Design review of the part built by this model. Coordinates are the model's own, in mm. Round coordinates to 2 decimals unless told otherwise and drop trailing zeros. Use a Markdown table: item, result.
from build123d import *

# Parameters (mm, degrees)
SKETCH1_W                        = 1212.85
SKETCH1_H                        = 584.2
BOSS_EXTRUDE1_DEPTH              = 3.175
SKETCH2_R                        = 5.3578125
SKETCH2_W                        = 63.5
SKETCH2_H                        = 88.9
CUT_EXTRUDE1_DEPTH               = 674.137439996
FILLET1_R                        = 6.35
SKETCH3_W                        = 142.875
SKETCH3_H                        = 88.9
CUT_EXTRUDE2_DEPTH               = 674.137439996
F_27_64_0_42188_DIAMETER_HOLE1_D = 10.715752
LPATTERN1_COUNT                  = 5
LPATTERN1_PITCH                  = 279.4
CUT_EXTRUDE3_DEPTH               = 674.137439996


with BuildPart() as part:
    # Sketch1 → Boss-Extrude1 (new, symmetric)
    with BuildSketch(Plane.XY):
        Rectangle(SKETCH1_W, SKETCH1_H)
    extrude(amount=BOSS_EXTRUDE1_DEPTH, both=True)

    # Sketch2 → Cut-Extrude1 (cut, through all)
    with BuildSketch(Plane.XY.offset(3.175)):
        with Locations((-466.725, 139.7)):
            Circle(SKETCH2_R)
        with Locations((-409.575, 139.7)):
            Circle(SKETCH2_R)
        with Locations((-466.725, -241.3)):
            Circle(SKETCH2_R)
        with Locations((-409.575, -241.3)):
            Circle(SKETCH2_R)
        with Locations((412.75, 139.7)):
            Circle(SKETCH2_R)
        with Locations((463.55, 139.7)):
            Circle(SKETCH2_R)
        with Locations((412.75, -241.3)):
            Circle(SKETCH2_R)
        with Locations((463.55, -241.3)):
            Circle(SKETCH2_R)
        with Locations((438.15, 247.65)):
            Rectangle(SKETCH2_W, SKETCH2_H)
        with Locations((-438.15, 247.65)):
            Rectangle(SKETCH2_W, SKETCH2_H)
    extrude(amount=-CUT_EXTRUDE1_DEPTH, mode=Mode.SUBTRACT)

    # Fillet1
    fillet1_edges = [part.edges().sort_by_distance(p)[0] for p in [
        (-406.4, 203.2, 0),
        (-469.9, 203.2, 0),
        (469.9, 203.2, 0),
        (406.4, 203.2, 0),
    ]]
    fillet(fillet1_edges, radius=FILLET1_R)

    # Sketch3 → Cut-Extrude2 (cut, through all)
    with BuildSketch(Plane.XY.offset(3.175)):
        with Locations((534.9875, 247.65)):
            Rectangle(SKETCH3_W, SKETCH3_H)
    extrude(amount=-CUT_EXTRUDE2_DEPTH, mode=Mode.SUBTRACT)

    # 27/64 (0.42188) Diameter Hole1 (through all)
    with Locations(Plane.XY.offset(3.175)):
        with Locations((-561.975, -280.9875)):
            f_27_64_0_42188_diameter_hole1 = Hole(F_27_64_0_42188_DIAMETER_HOLE1_D / 2)

    # LPattern1: 27/64 (0.42188) Diameter Hole1 ×5
    with Locations(*[(i * LPATTERN1_PITCH, 0, 0) for i in range(1, LPATTERN1_COUNT)]):
        add(f_27_64_0_42188_diameter_hole1, mode=Mode.SUBTRACT)

    # Sketch6 → Cut-Extrude3 (cut, through all)
    with BuildSketch(Plane.XY.offset(3.175)):
        with BuildLine():
            Line((-606.425, 292.1), (-606.425, 266.7))
            Line((-606.425, 266.7), (-536.575, 266.7))
            ThreePointArc((-536.575, 266.7), (-532.084871939, 268.559871939), (-530.225, 273.05))
            Line((-530.225, 273.05), (-530.225, 292.1))
            Line((-530.225, 292.1), (-606.425, 292.1))
        make_face()
    extrude(amount=-CUT_EXTRUDE3_DEPTH, mode=Mode.SUBTRACT)


solid = part.part
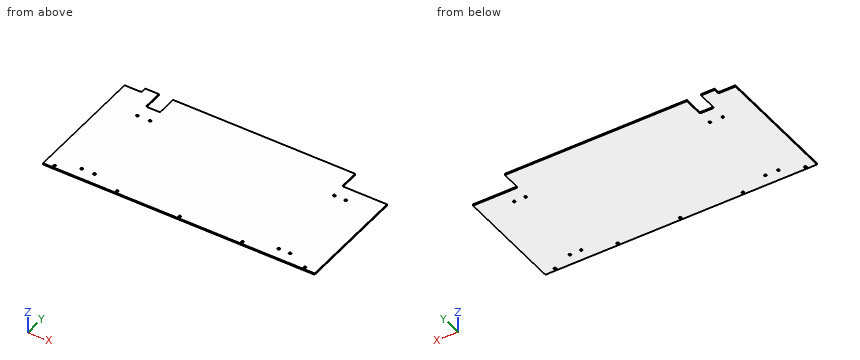
1. Wall thickness on line 1 along X through (y, z) = (257.5, -2.25) (3 decimals): over which ranges is the line inside the solid? List them lowest first. Write a range as from..to.
Check values:
| item | result |
|---|---|
| line 1 | x = -606.425..-469.9, -406.4..406.4 |
2. Take a section at A-A on z = 0. Count the separate pieces of the cut face and the enclosed holes in it, and give its area (3 significant figures).
Check values:
| item | result |
|---|---|
| separate pieces | 1 |
| enclosed holes | 13 |
| area | 682,000 mm² |
3. Insertion check: pin 1 (9.5 mm diameter, centred on x = 412.75, y = 139.7, fed in from +Z); pin 2 (1.9 mm diameter, centred on y = 271.5, z = 1, fed in from +X); pin 3 (3 mm diameter, centred on x = 413.5, z = 1, fed in from +Y). Each pin has a flat end and moves straight along its axis. Give the tip position at first contact, or say it passes through.
Check values:
| item | result |
|---|---|
| pin 1 | passes through |
| pin 2 | stops at x = 406.4 |
| pin 3 | stops at y = 203.24 |
